```python
from build123d import *

# Parameters (mm, degrees)
SKETCH4_W                = 12.46
SKETCH4_H                = 17.25
BOSS_EXTRUDE3_DEPTH      = 6
SKETCH8_R                = 12.546781182
SKETCH8_R_2              = 11.15
BOSS_EXTRUDE6_DEPTH      = 7.3
BOSS_EXTRUDE6_DEPTH_BACK = 17.25
BOSS_EXTRUDE4_DEPTH      = 17.25
SKETCH6_R                = 0.5
CUT_EXTRUDE1_DEPTH       = 15
CHAMFER1_SIZE            = 0.5
CHAMFER1_SIZE2           = 0.866025404
SKETCH10_W               = 12.46
SKETCH10_H               = 23.7
CUT_EXTRUDE3_DEPTH       = 17.25
CUT_EXTRUDE4_REACH       = 38.097
SKETCH11_W               = 5
SKETCH11_H               = 3
BOSS_EXTRUDE7_DEPTH      = 7.3
BOSS_EXTRUDE9_DEPTH      = 10
SKETCH20_R               = 11.15
SKETCH20_R_2             = 7.15
BOSS_EXTRUDE11_DEPTH     = 7.3
SKETCH21_R               = 10.15
SKETCH21_R_2             = 7.15
CUT_EXTRUDE7_DEPTH       = 1.3
BOSS_EXTRUDE10_DEPTH     = 25.093562
SKETCH18_W               = 20
SKETCH18_H               = 12.438292938
CUT_EXTRUDE5_DEPTH       = 2
SKETCH19_R               = 1.25
CUT_EXTRUDE6_DEPTH       = 53.75
CUT_EXTRUDE6_DEPTH_BACK  = 3
FILLET1_R                = 10
SKETCH22_R               = 5.8
BOSS_EXTRUDE12_DEPTH     = 20
FILLET2_R                = 2
SKETCH23_R               = 5.930854157
SKETCH23_R_2             = 5.08
CUT_EXTRUDE8_DEPTH       = 11.6
SKETCH24_R               = 6.5
BOSS_EXTRUDE13_DEPTH     = 2
SKETCH25_R               = 1.25
BOSS_EXTRUDE14_DEPTH     = 2
SKETCH26_W               = 5
SKETCH26_H               = 3
BOSS_EXTRUDE15_DEPTH     = 5


with BuildPart() as part:
    # Sketch4 → Boss-Extrude3 (new body)
    with BuildSketch(Plane.XY):
        with Locations((0, -1.35)):
            Rectangle(SKETCH4_W, SKETCH4_H)
    extrude(amount=BOSS_EXTRUDE3_DEPTH)



with BuildPart() as body_2:
    # Sketch8 → Boss-Extrude6 (new body, two sides)
    with BuildSketch(Plane(origin=(0, -9.975, 0), x_dir=(-1, 0, 0), z_dir=(0, -1, 0))) as boss_extrude6_sk:
        with Locations((0, -23.55)):
            Circle(SKETCH8_R)
        with Locations((0, -23.55)):
            Circle(SKETCH8_R_2, mode=Mode.SUBTRACT)
    extrude(amount=BOSS_EXTRUDE6_DEPTH)
    extrude(boss_extrude6_sk.sketch, amount=-BOSS_EXTRUDE6_DEPTH_BACK)


with BuildPart() as part_1:
    add(part.part)

    add(body_2.part)  # Boss-Extrude4 merges body 2
    # Sketch5 → Boss-Extrude4 (add)
    with BuildSketch(Plane(origin=(0, 7.275, 0), x_dir=(1, 0, 0), z_dir=(0, 1, 0))):
        with BuildLine():
            Line((12.546781182, -23.55), (12.546781182, 0))
            Line((12.546781182, 0), (6.23, 0))
            Line((6.23, 0), (6.23, -29.7))
            Line((6.23, -29.7), (-6.23, -29.7))
            Line((-6.23, -29.7), (-6.23, 0))
            Line((-6.23, 0), (-12.546781182, 0))
            Line((-12.546781182, 0), (-12.546781182, -23.55))
            ThreePointArc((-12.546781182, -23.55), (0, -36.096781182), (12.546781182, -23.55))
        make_face()
    extrude(amount=-BOSS_EXTRUDE4_DEPTH)

    # Sketch6 → Cut-Extrude1 (cut)
    with BuildSketch(Plane(origin=(0, 7.275, 0), x_dir=(1, 0, 0), z_dir=(0, 1, 0))):
        with Locations((0, -3.6)):
            Circle(SKETCH6_R)
        with Locations((0, -32.1)):
            Circle(SKETCH6_R)
    extrude(amount=-CUT_EXTRUDE1_DEPTH, mode=Mode.SUBTRACT)

    # Chamfer1
    chamfer1_edges = [part_1.edges().sort_by_distance(p)[0] for p in [
        (-0.5, 7.275, 3.6),
        (-0.5, 7.275, 32.1),
    ]]
    chamfer1_side = [part_1.faces().sort_by_distance(p)[0] for p in [
        (0, 7.275, 35.657160381),
    ]]
    chamfer(chamfer1_edges, length=CHAMFER1_SIZE, length2=CHAMFER1_SIZE2, reference=chamfer1_side[0])

    # Sketch10 → Cut-Extrude3 (cut)
    with BuildSketch(Plane(origin=(0, 7.275, 0), x_dir=(1, 0, 0), z_dir=(0, 1, 0))):
        with Locations((0, -17.85)):
            Rectangle(SKETCH10_W, SKETCH10_H)
    extrude(amount=-CUT_EXTRUDE3_DEPTH, mode=Mode.SUBTRACT)

    # Sketch11 → Cut-Extrude4 (cut, up to next)
    with BuildSketch(Plane.XY.offset(36.096781182), mode=Mode.PRIVATE) as cut_extrude4_sk1:
        with Locations((0, -8.475)):
            Rectangle(SKETCH11_W, SKETCH11_H)
    cut_extrude4_tool1 = extrude(cut_extrude4_sk1.sketch, amount=-CUT_EXTRUDE4_REACH, mode=Mode.PRIVATE) & part_1.part
    add(cut_extrude4_tool1.solids().sort_by_distance((0, -8.475, 36.096781))[0], mode=Mode.SUBTRACT)

    # Sketch13 → Boss-Extrude7 (add)
    with BuildSketch(Plane.XZ.offset(17.275)):
        with BuildLine():
            Line((-12.546781182, 23.55), (-12.546781182, 0))
            Line((-12.546781182, 0), (12.546781182, 0))
            Line((12.546781182, 0), (12.546781182, 23.55))
            ThreePointArc((12.546781182, 23.55), (0, 11.003218818), (-12.546781182, 23.55))
        make_face()
    extrude(amount=-BOSS_EXTRUDE7_DEPTH)

    # Sketch15 → Boss-Extrude9 (add)
    with BuildSketch(Plane(origin=(0, 7.275, 0), x_dir=(1, 0, 0), z_dir=(0, 1, 0))):
        with BuildLine():
            Line((-12.546781182, 0), (12.546781182, 0))
            Line((12.546781182, 0), (12.546781182, -23.55))
            ThreePointArc((12.546781182, -23.55), (0, -36.096781182), (-12.546781182, -23.55))
            Line((-12.546781182, -23.55), (-12.546781182, 0))
        make_face()
        with BuildLine():
            Line((-6.23, -0.8), (6.23, -0.8))
            Line((6.23, -0.8), (6.23, -33.5))
            ThreePointArc((6.23, -33.5), (5.937106781, -34.207106781), (5.23, -34.5))
            Line((5.23, -34.5), (-5.23, -34.5))
            ThreePointArc((-5.23, -34.5), (-5.937106781, -34.207106781), (-6.23, -33.5))
            Line((-6.23, -33.5), (-6.23, -0.8))
        make_face(mode=Mode.SUBTRACT)
    extrude(amount=BOSS_EXTRUDE9_DEPTH)

    # Sketch20 → Boss-Extrude11 (add)
    with BuildSketch(Plane.XZ.offset(17.275)):
        with Locations((0, 23.55)):
            Circle(SKETCH20_R)
        with Locations((0, 23.55)):
            Circle(SKETCH20_R_2, mode=Mode.SUBTRACT)
    extrude(amount=-BOSS_EXTRUDE11_DEPTH)

    # Sketch21 → Cut-Extrude7 (cut)
    with BuildSketch(Plane.XZ.offset(17.275)):
        with Locations((0, 23.55)):
            Circle(SKETCH21_R)
        with Locations((0, 23.55)):
            Circle(SKETCH21_R_2, mode=Mode.SUBTRACT)
    extrude(amount=-CUT_EXTRUDE7_DEPTH, mode=Mode.SUBTRACT)

    # Sketch17 → Boss-Extrude10 (add)
    with BuildSketch(Plane(origin=(12.546781182, 4.728218818, 0), x_dir=(0, 1, 0), z_dir=(-1, 0, 0))):
        Polygon((16.946781182, 25), (16.946781182, 0), (-37.803218818, 0), (-37.803218818, 25), (-33.803218818, 25), (-33.803218818, 5), (12.946781182, 5), (12.946781182, 25), align=None)
    extrude(amount=BOSS_EXTRUDE10_DEPTH)

    # Sketch18 → Cut-Extrude5 (cut)
    with BuildSketch(Plane(origin=(0, 17.675, 0), x_dir=(0, 0, 1), z_dir=(0, -1, 0))):
        with Locations((-15, 0)):
            Rectangle(SKETCH18_W, SKETCH18_H)
    extrude(amount=-CUT_EXTRUDE5_DEPTH, mode=Mode.SUBTRACT)

    # Sketch19 → Cut-Extrude6 (cut, two sides)
    with BuildSketch(Plane(origin=(0, 19.675, 0), x_dir=(0, 0, 1), z_dir=(0, -1, 0))) as cut_extrude6_sk:
        with Locations((-20, 0)):
            Circle(SKETCH19_R)
    extrude(amount=CUT_EXTRUDE6_DEPTH, mode=Mode.SUBTRACT)
    extrude(cut_extrude6_sk.sketch, amount=-CUT_EXTRUDE6_DEPTH_BACK, mode=Mode.SUBTRACT)

    # Fillet1
    fillet1_edges = [part_1.edges().sort_by_distance(p)[0] for p in [
        (-12.546780818, 19.675, -25),
        (12.546781182, 19.675, -25),
        (-12.546780818, -31.075, -25),
        (12.546781182, -31.075, -25),
    ]]
    fillet(fillet1_edges, radius=FILLET1_R)

    # Sketch22 → Boss-Extrude12 (add)
    with BuildSketch(Plane(origin=(0, -29.075, 0), x_dir=(0, 0, -1), z_dir=(0, 1, 0))):
        with Locations((20, 0)):
            Circle(SKETCH22_R)
    extrude(amount=BOSS_EXTRUDE12_DEPTH)

    # Fillet2
    fillet2_edges = [part_1.edges().sort_by_distance(p)[0] for p in [
        (0, -9.075, -14.2),
    ]]
    fillet(fillet2_edges, radius=FILLET2_R)

    # Sketch23 → Cut-Extrude8 (cut)
    with BuildSketch(Plane(origin=(0, -29.075, 0), x_dir=(0, 0, -1), z_dir=(0, 1, 0))):
        with Locations((20, 0)):
            Circle(SKETCH23_R)
        with Locations((20, 0)):
            Circle(SKETCH23_R_2, mode=Mode.SUBTRACT)
    extrude(amount=CUT_EXTRUDE8_DEPTH, mode=Mode.SUBTRACT)

    # Sketch24 → Boss-Extrude13 (add)
    with BuildSketch(Plane(origin=(0, -17.475, 0), x_dir=(0, 0, 1), z_dir=(0, -1, 0))):
        with Locations((-20, 0)):
            Circle(SKETCH24_R)
    extrude(amount=BOSS_EXTRUDE13_DEPTH)

    # Sketch25 → Boss-Extrude14 (add)
    with BuildSketch(Plane(origin=(0, -33.075, 0), x_dir=(0, 0, 1), z_dir=(0, -1, 0))):
        with Locations((-20, 0)):
            Circle(SKETCH25_R)
    extrude(amount=-BOSS_EXTRUDE14_DEPTH)

    # Sketch26 → Boss-Extrude15 (add)
    with BuildSketch(Plane(origin=(0, -29.075, 0), x_dir=(0, 0, -1), z_dir=(0, 1, 0))):
        with Locations((7.5, -8.296781182)):
            Rectangle(SKETCH26_W, SKETCH26_H)
        with Locations((7.5, -3.780781182)):
            Rectangle(SKETCH26_W, SKETCH26_H)
    extrude(amount=BOSS_EXTRUDE15_DEPTH)


solid = part_1.part
```
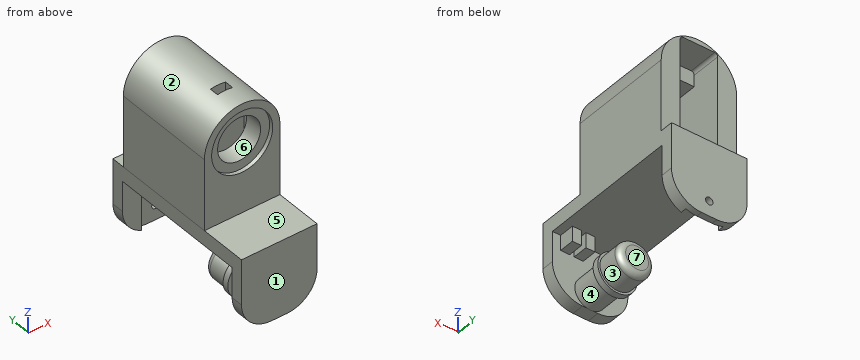
Model file for the job. Use its own axes, mm. Face numbers are marked on the shaded views. A direction names the side the tool comes from. Coordinates: 2 decimals unless noted, no trailing zeros. Write each loop counter-clockwise with the first axis right and the second up, starting at its lowest first coordinate (ties: lowest second). Pieces come first, ordered by that corner, then holes. Notation, with made-up numbers: (50.5, -19.75) - (106.5, -19.75) arc R10 cw to (106.5, -5.75) - close; hole circle Ø5 at (88.25, 46.25). An arc over 180 degrees is marked (long way). One line per item, written item: value. Start each with the question number.
1. Slice it at A-A (y = -25). Write the cut outline in (x, z), plus the area to 3 significant figures.
2. Flat gauge pins, fed straight in: pin 1 (2 mm diameter, centred on x = 0, z = -20, fed in from +Y) (3 decimals); pin 2 (2 mm diameter, centred on x = 6, y = 5.5, fed in from -Z); pin 3 (3 mm diameter, centred on x = -6.5, z = 18, fed in from -Y) (3 decimals); pin 4 (6 mm diameter, centred on x = 1, z = 20.5, fed in from -Y). Where does each tip first touch, or does it go through?
3. Slice it at D-D (z = 25.5). Write the cut outline in (x, y) (3 decimals).
4. Slice it at C-C (y = 8.5). Write the cut outline in (x, z), plus the area to 3 significant figures.
5. Tool access for the marked faces 4, 5, 6 and 7: list every direction of +Z, -Z, +X, -X, +Y, -Y with a clear straight run to the whole face (end or side of a thin tool).
6. Slice it at B-B (z = -20). Count the separate pieces of the cut face and the enclosed holes in it, plus the area to 3 significant figures.
7. Probe line 1 (Z direction, x = 0, y = -12.5); line 2 (Z direction, x = 0, y = -2.5); line 3 (Y direction, x = 3, z = -13) (3 decimals). List the from-to ranges inside material, lowest first. Write a range as from..to.
8. Mould opens along Z. For the marked faces 1, 2 and 3 say: released by +Z, released by -Z, zero draft, split by the parting line, or undercut.
Answers below:
1. outline: (-12.55, -5) - (2.28, -5) - (2.28, -10) - (5.28, -10) - (5.28, -5) - (6.8, -5) - (6.8, -10) - (9.8, -10) - (9.8, -5) - (12.55, -5) - (12.55, 0) - (-12.55, 0) - close; circle Ø10.16 at (0, -20)
1. area: 237 mm^2
2. pin 1: stops at y = -9.075
2. pin 2: stops at z = -5
2. pin 3: stops at y = -15.975
2. pin 4: passes through
3. outline: (-12.394, -17.275) - (-9.961, -17.275) - (-9.961, -15.975) - (-6.879, -15.975) - (-6.879, -9.975) - (-6.23, -9.975) - (-6.23, 17.275) - (-12.394, 17.275) - close; (6.23, -9.975) - (6.879, -9.975) - (6.879, -15.975) - (9.961, -15.975) - (9.961, -17.275) - (12.394, -17.275) - (12.394, 17.275) - (6.23, 17.275) - close
4. outline: (-12.55, -5) - (12.55, -5) - (12.55, 23.55) arc R12.55 ccw to (-12.55, 23.55) - close; hole (-6.23, 0.8) - (6.23, 0.8) - (6.23, 33.5) arc R1 ccw to (5.23, 34.5) - (-5.23, 34.5) arc R1 ccw to (-6.23, 33.5) - close
4. area: 544 mm^2
5. face 4: none
5. face 5: +Z, +X, -X, -Y
5. face 6: -Y
5. face 7: -Z, +X, -X
6. separate pieces: 3
6. enclosed holes: 1
6. area: 364 mm^2
7. line 1: z = -25.8..-14.2, -5..16.4, 30.7..36.1
7. line 2: z = -5..3.1, 4.1..6, 29.7..31.6, 32.6..36.1
7. line 3: y = -33.075..-29.075, 19.675..21.675
8. face 1: zero draft
8. face 2: released by +Z
8. face 3: undercut
